CAD build for the part. Positions are in the model's coordinates, mm. Give positions to 0.01 mm unless a question says otherwise; leave off trailing zeros. Loops run counter-clockwise (first coordinate to the right, second up) from the corner with the lowest first, then second, coordinate; pieces in that order, holes last.
Item 1: Saw through at B-B on x = 0. Give the cut face in (y, z).
Item 2: Saw through at D-D on z = 0.25. Give the cut face in (x, y), plus the area to 3 significant figures.
Item 3: Probe probe 1 along X at (y, z) = (-9, 0.95); probe 2 along X at (y, z) = (2, 0.3); probe 3 along Y at (x, z) = (2.5, 0.5). List the from-to ranges inside material, lowest first.
Item 4: Saw through at A-A on y = 24. Give the cut face in (x, z).
Item 5: Saw through at C-C on y = -28. Give the cut face in (x, z).
Item 6: Drop a flat-ended pin along its axis: P1, Ø21, axis at x = 0, y = -1.96, coming from the +Z side. Give the stop position or say it passes through.
from build123d import *

# Parameters (mm, degrees)
F0_R     = 15
F0_R_2   = 14
F0_R_3   = 13
F0_R_4   = 16
F0_R_5   = 12
F0_R_6   = 18
F0_R_7   = 17
F1_DEPTH = 1


with BuildPart() as f1:
    # F0 (on Top) → F1 (new body)
    with BuildSketch(Plane.XY):
        with BuildLine():
            Line((-16, -47.370877), (16, -47.370877))
            ThreePointArc((16, -47.370877), (0, 50), (-16, -47.370877))
        make_face()
        with Locations((-9.797097, -30.697571)):
            Circle(F0_R, mode=Mode.SUBTRACT)
        with Locations((-33.496745, -10.543544)):
            Circle(F0_R_2, mode=Mode.SUBTRACT)
        with Locations((0, -1.95942)):
            Circle(F0_R_3, mode=Mode.SUBTRACT)
        with Locations((21.740226, -23.606339)):
            Circle(F0_R_4, mode=Mode.SUBTRACT)
        with Locations((-29.764516, 17.448165)):
            Circle(F0_R_5, mode=Mode.SUBTRACT)
        with Locations((0, 30.884182)):
            Circle(F0_R_6, mode=Mode.SUBTRACT)
        with Locations((30.137738, 9.797097)):
            Circle(F0_R_7, mode=Mode.SUBTRACT)
    extrude(amount=F1_DEPTH)


solid = f1.part
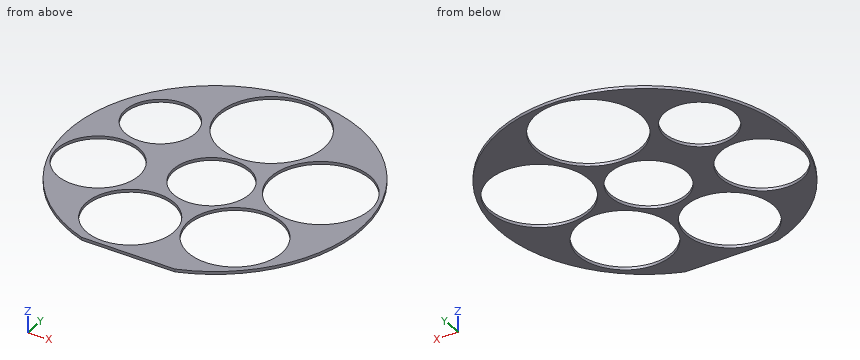
Results below:
1. outline: (-47.37, 0) - (-42.06, 0) - (-42.06, 1) - (-47.37, 1) - close; (-19.34, 0) - (-14.96, 0) - (-14.96, 1) - (-19.34, 1) - close; (11.04, 0) - (12.88, 0) - (12.88, 1) - (11.04, 1) - close; (48.88, 0) - (50, 0) - (50, 1) - (48.88, 1) - close
2. outline: (-16, -47.37) - (16, -47.37) arc R50 ccw (long way) to start; hole circle Ø28 at (-33.5, -10.54); hole circle Ø24 at (-29.76, 17.45); hole circle Ø30 at (-9.8, -30.7); hole circle Ø36 at (0, 30.88); hole circle Ø26 at (0, -1.96); hole circle Ø32 at (21.74, -23.61); hole circle Ø34 at (30.14, 9.8)
2. area: 2,760 mm2
3. probe 1: x = -49.18 to -47.41, -19.58 to -10.93, 10.93 to 15.21, 28.27 to 49.18
3. probe 2: x = -49.96 to -39.71, -27.28 to -12.38, 12.38 to 15.03, 45.24 to 49.96
3. probe 3: y = -47.37 to -39.29, -22.11 to -14.72, 10.8 to 13.06, 48.71 to 49.94
4. outline: (-43.86, 0) - (-39.82, 0) - (-39.82, 1) - (-43.86, 1) - close; (-19.71, 0) - (-16.63, 0) - (-16.63, 1) - (-19.71, 1) - close; (16.63, 0) - (20.8, 0) - (20.8, 1) - (16.63, 1) - close; (39.48, 0) - (43.86, 0) - (43.86, 1) - (39.48, 1) - close
5. outline: (-41.42, 0) - (-24.55, 0) - (-24.55, 1) - (-41.42, 1) - close; (4.96, 0) - (6.36, 0) - (6.36, 1) - (4.96, 1) - close; (37.13, 0) - (41.42, 0) - (41.42, 1) - (37.13, 1) - close
6. P1: passes through
